from build123d import *

# Parameters (mm, degrees)
BOSS_EXTRUDE1_DEPTH = 70
SKETCH3_W           = 4
SKETCH3_H           = 30
BOSS_EXTRUDE2_DEPTH = 10
CUT_EXTRUDE1_DEPTH  = 168
FILLET2_R           = 3
FILLET3_R           = 2
FILLET4_R           = 30


with BuildPart() as part:
    # Sketch1 → Boss-Extrude1 (new body)
    with BuildSketch(Plane(origin=(0, 0, 0), x_dir=(1, 0, 0), z_dir=(0, 1, 0))):
        with BuildLine():
            Line((-78, 0), (-76, 0))
            ThreePointArc((-76, 0), (0, 43.107230832), (76, 0))
            Line((76, 0), (78, 0))
            ThreePointArc((78, 0), (0, 45.008730356), (-78, 0))
        make_face()
    extrude(amount=BOSS_EXTRUDE1_DEPTH)

    # Sketch3 → Boss-Extrude2 (add)
    with BuildSketch(Plane.XY):
        with Locations((-78, 15)):
            Rectangle(SKETCH3_W, SKETCH3_H)
        with Locations((78, 15)):
            Rectangle(SKETCH3_W, SKETCH3_H)
    extrude(amount=BOSS_EXTRUDE2_DEPTH)

    # Sketch4 → Cut-Extrude1 (cut)
    with BuildSketch(Plane.ZY.offset(80)):
        with BuildLine():
            Line((7.1, 25.7), (7.1, 4.3))
            ThreePointArc((7.1, 4.3), (5, 2.2), (2.9, 4.3))
            Line((2.9, 4.3), (2.9, 25.7))
            ThreePointArc((2.9, 25.7), (5, 27.8), (7.1, 25.7))
        make_face()
    extrude(amount=-CUT_EXTRUDE1_DEPTH, mode=Mode.SUBTRACT)

    # Fillet2
    fillet2_edges = [part.edges().sort_by_distance(p)[0] for p in [
        (-78, 15, 0),
        (-78, 30, 10),
        (-78, 0, 10),
        (78, 0, 10),
        (78, 30, 10),
        (78, 15, 0),
    ]]
    fillet(fillet2_edges, radius=FILLET2_R)

    # Fillet3
    fillet3_edges = [part.edges().sort_by_distance(p)[0] for p in [
        (-77, 30, 0),
        (77, 30, 0),
    ]]
    fillet(fillet3_edges, radius=FILLET3_R)

    # Fillet4
    # the kernel refuses this fillet: 30 mm, written as the material it takes off along each edge
    with BuildSketch(Plane(origin=(-153, 70, 0), x_dir=(0, 0, -1), z_dir=(1, 0, 0))) as fillet4_piece_1:
        with BuildLine():
            CenterArc((FILLET4_R, -FILLET4_R), FILLET4_R, 90, 90)
            Line((0, -FILLET4_R), (0, 0))
            Line((0, 0), (FILLET4_R, 0))
        make_face()
    extrude(amount=152, mode=Mode.SUBTRACT)
    with BuildSketch(Plane(origin=(1, 70, 0), x_dir=(0, -1, 0), z_dir=(1, 0, 0))) as fillet4_piece_2:
        with BuildLine():
            CenterArc((FILLET4_R, FILLET4_R), FILLET4_R, 180, 90)
            Line((0, FILLET4_R), (0, 0))
            Line((0, 0), (FILLET4_R, 0))
        make_face()
    extrude(amount=152, mode=Mode.SUBTRACT)


solid = part.part
For this review, take the finished solid that the model builds, in its own axes (mm). A direction names the side the tool comes from. Round coordinates to 2 decimals unless told otherwise and drop trailing zeros. Write each loop counter-clockwise with the first axis right and the second up, starting at its lowest first coordinate (ties: lowest second). Pieces come first, ordered by that corner, then holes. Notation, with made-up numbers: (5.5, 22) - (17.5, 22) arc R15 cw to (17.5, 34) - close; hole circle Ø10 at (-9, 33). An arc over 180 degrees is marked (long way). Write item = value, one per line. Start each with the question number.
1. Consider section C-C on z = -15. State the section outline as (x, y) points.
2. Consider section A-A on y = 21. State the section outline as (x, z) points, plus the area to 3 significant figures.
3. Consider section B-B on z = 5. State the section outline as (x, y) points.
4. Wall thickness on L1, parallel to X at y = 26, z = -34; L2, parallel to X at y = 41, z = -31; L3, parallel to Z at x = 19, y = 57: over which ranges is each line inside the solid? List them lowest first.
5. For faces 1 (the face through (-78, 15, 10)), 2 (the face through (78, 15, 2.9)), list the 3-axis set-ups (+Z, -Z, +X, -X, +Y, -Y) from which the entire face can be reached by the end or side of a thin tool; tool diameter is ignored.
6. Consider section D-D on y = 35. State the section outline as (x, z) points.
7. For pin 1 Ø1.2 at (x, z) = (-78.5, 4) entering from +Y; pin 2 Ø3 at (x, y) = (-78.5, 16.5) entering from -Z; pin 3 Ø1.2 at (x, z) = (79, 1.5) entering from +Y, all flat-tipped, find the tip position at first contact; note any pin that passes through.
Evaluation:
q1.outline = (-67.13, 0) - (-64.71, 0) - (-64.71, 65.98) - (-67.13, 65.98) - close; (64.71, 0) - (67.13, 0) - (67.13, 65.98) - (64.71, 65.98) - close
q2.outline = (-80, 0) - (-79.71, 0) arc R3 cw to (-77.14, -1.45) arc R90.09 ccw to (77.14, -1.45) arc R3 cw to (79.71, 0) - (80, 0) - (80, 2.9) - (76, 2.9) - (76, 0) arc R88.55 cw to (-76, 0) - (-76, 2.9) - (-80, 2.9) - close; (-80, 7.1) - (-76, 7.1) - (-76, 10) - (-80, 10) - close; (76, 7.1) - (80, 7.1) - (80, 10) - (76, 10) - close
q2.area = 389 mm2
q3.outline = (-80, 0) - (-76, 0) - (-76, 2.2) - (-80, 2.2) - close; (-80, 27.8) - (-76, 27.8) - (-76, 30) - (-80, 30) - close; (76, 0) - (80, 0) - (80, 2.2) - (76, 2.2) - close; (76, 27.8) - (80, 27.8) - (80, 30) - (76, 30) - close
q4.L1 = -43.16 to -39.11, 39.11 to 43.16
q4.L2 = -48.25 to -44.69, 44.69 to 48.25
q4.L3 = -42.98 to -41.04
q5.face_1 = +Z, +X, -X, +Y, -Y
q5.face_2 = +X, -X
q6.outline = (-78, 0) arc R90.09 ccw to (78, 0) - (76, 0) arc R88.55 cw to (-76, 0) - close
q7.pin_1 = 30
q7.pin_2 = -1.69
q7.pin_3 = 30.24
